Model file for the job. Use its own axes, mm. Face numbers are marked on the shaded views. A direction names the side the tool comes from. Coordinates: 2 decimals unless noted, no trailing zeros. Loops run counter-clockwise (first coordinate to the right, second up) from the corner with the lowest first, then second, coordinate; pieces in that order, holes last. Notation, with made-up numbers: (-33, 36.5) -> (6, 36.5) arc R16 cw to (6, 45.5) -> close; hole circle Ø4 at (32, 64). An arc over 180 degrees is marked (long way). Use one line per item in the form item = value.
```python
from build123d import *

# Parameters (mm, degrees)
F0_R     = 3
F1_DEPTH = 14
F3_DEPTH = 3


with BuildPart() as f1:
    # F0 (on Front) → F1 (new body)
    with BuildSketch(Plane.XZ):
        Circle(F0_R)
    extrude(amount=F1_DEPTH)

    # F2 (on face) → F3 (join)
    with BuildSketch(Plane(origin=(0, 0, 0), x_dir=(-1, 0, 0), z_dir=(0, 1, 0))):
        with BuildLine():
            ThreePointArc((-10, 0), (-9.1213203436, -2.1213203436), (-7, -3))
            Line((-7, -3), (0, -3))
            ThreePointArc((0, -3), (-3, 0), (0, 3))
            Line((0, 3), (-7, 3))
            ThreePointArc((-7, 3), (-9.1213203436, 2.1213203436), (-10, 0))
        make_face()
        with BuildLine():
            ThreePointArc((3, 0), (2.1213203436, -2.1213203436), (0, -3))
            Line((0, -3), (7, -3))
            ThreePointArc((7, -3), (9.1213203436, -2.1213203436), (10, 0))
            ThreePointArc((10, 0), (9.1213203436, 2.1213203436), (7, 3))
            Line((7, 3), (0, 3))
            ThreePointArc((0, 3), (2.1213203436, 2.1213203436), (3, 0))
        make_face()
        with BuildLine():
            ThreePointArc((0, 3), (-3, 0), (0, -3))
            ThreePointArc((0, -3), (2.1213203436, -2.1213203436), (3, 0))
            ThreePointArc((3, 0), (2.1213203436, 2.1213203436), (0, 3))
        make_face()
    extrude(amount=F3_DEPTH)


solid = f1.part
```
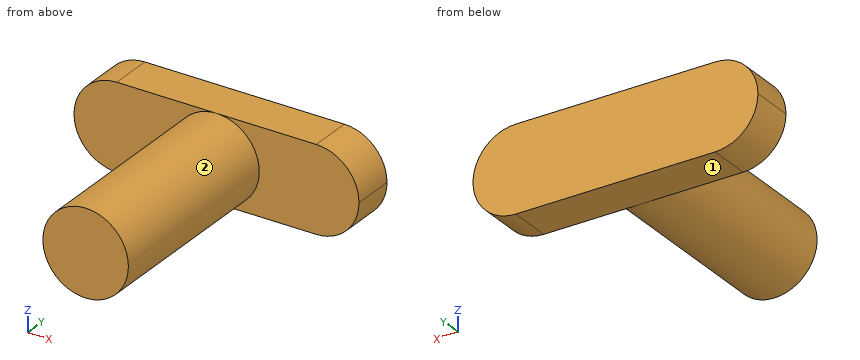
Q1. Band-saw the part on C-C, the plane x = 4.25. Write the cut outline in (y, z), and give its area (3 significant figures).
Result:
outline = (0, -3) -> (3, -3) -> (3, 3) -> (0, 3) -> close
area = 18.0 mm2
Q2. Which spindle directions (+Z, -Z, +X, -X, +Y, -Y) get a long thin tool onto all of the face, cutting with end or side? Do the marked faces 1 and 2. Say none if no direction does.
Result:
face_1 = -Z, +X, -X, +Y, -Y
face_2 = -Y
Q3. Band-saw the part on A-A, the plane z = 1.2. Write the cut outline in (x, y), and give its area (3 significant figures).
Result:
outline = (-9.75, 0) -> (-2.75, 0) -> (-2.75, -14) -> (2.75, -14) -> (2.75, 0) -> (9.75, 0) -> (9.75, 3) -> (-9.75, 3) -> close
area = 135 mm2
Q4. Wall check: line 1 along Y through (x, z) = (-4.25, -0.4); line 2 along X through (y, z) = (-3.25, 0); line 3 along X through (y, z) = (-6, 1.15). Give the ranges that are in metal, low to high.
Result:
line_1 = 0 to 3
line_2 = -3 to 3
line_3 = -2.77 to 2.77
Q5. Pin check, flat tips, straight feed: pin 1 Ø3 at (y, z) = (-12, 1) entering from +X; pin 2 Ø1.5 at (x, y) = (4, -11) entering from +Z; pin 3 Ø1 at (y, z) = (-7.5, 2) entering from -X; pin 4 Ø3 at (y, z) = (-8.5, -2) entering from -X. Stop position of each tip, or through.
Result:
pin_1 = 3
pin_2 = through
pin_3 = -2.6
pin_4 = -2.96
Q6. Band-saw the part on D-D, the plane z = -2.15. Write the cut outline in (x, y).
Result:
outline = (-9.09, 0) -> (-2.09, 0) -> (-2.09, -14) -> (2.09, -14) -> (2.09, 0) -> (9.09, 0) -> (9.09, 3) -> (-9.09, 3) -> close
Q7. Band-saw the part on B-B, the plane y = -2. Write the cut outline in (x, z).
Result:
outline = circle Ø6 at (0, 0)
